from build123d import *

# Parameters (mm, degrees)
F0_W     = 380
F0_H     = 380
F1_DEPTH = 350
F2_W     = 342
F2_H     = 312
F3_DEPTH = 316
F4_W     = 40
F4_H     = 40
F5_DEPTH = 150


with BuildPart() as f1:
    # F0 (on Top) → F1 (new body)
    with BuildSketch(Plane.XY):
        Rectangle(F0_W, F0_H)
    extrude(amount=F1_DEPTH)

    # F2 (on face) → F3 (cut)
    with BuildSketch(Plane.XZ.offset(190)):
        with Locations((0, 175)):
            Rectangle(F2_W, F2_H)
    extrude(amount=-F3_DEPTH, mode=Mode.SUBTRACT)

    # F4 (on face) → F5 (join)
    with BuildSketch(Plane(origin=(0, 0, 0), x_dir=(1, 0, 0), z_dir=(0, 0, -1))):
        with Locations((170, 170)):
            Rectangle(F4_W, F4_H)
        with Locations((-170, -170)):
            Rectangle(F4_W, F4_H)
        with Locations((170, -170)):
            Rectangle(F4_W, F4_H)
        with Locations((-170, 170)):
            Rectangle(F4_W, F4_H)
    extrude(amount=F5_DEPTH)


solid = f1.part
The listing builds one solid part. Answer for the finished solid, in the listing's coordinates (mm). A direction names the side the tool comes from. Give positions to 0.01 mm unless a question says otherwise; leave off trailing zeros. Write each loop counter-clockwise with the first axis right and the second up, starting at its lowest first coordinate (ties: lowest second). Pieces come first, ordered by that corner, then holes. Notation, with made-up numbers: (70, -1) -> (107, -1) arc R11 ccw to (107, 14) -> close; hole circle Ø3 at (41.5, 58.25). An arc over 180 degrees is marked (long way). Use a Markdown table: item, result.
(1) Section C-C, the plane z = 247 is taken. Determine the outline of the cut face in (x, y), then the cut area to 3 significant figures.
Return value:
| item | result |
|---|---|
| outline | (-190, -190) -> (-171, -190) -> (-171, 126) -> (171, 126) -> (171, -190) -> (190, -190) -> (190, 190) -> (-190, 190) -> close |
| area | 36,300 mm2 |
(2) Determine the mould class of faces 6 (the flat face through (-170, -150, -74)), 7 (the flat face through (-170, 150, -74)), 8 (the flat face through (-190, -3, 152)), 9 (the flat face through (-3, 190, 152)) for opening direction Y: released by +Y, released by -Y, zero draft, split by the parting line, or undercut.
Return value:
| item | result |
|---|---|
| face 6 | undercut |
| face 7 | undercut |
| face 8 | zero draft |
| face 9 | released by +Y |
(3) A flat-ended cylindrical pin translates along its axis: P1, Ø6, axis at x = 33.5, y = 118.5, coming from the -Z side. Find the tip coordinate at first contact, or state that the pin passes through.
Return value:
| item | result |
|---|---|
| P1 | z = 0 |
(4) Find the intervals of material crossed by probe 1 along X at (y, z) = (-19, 20); probe 2 along Z at (x, y) = (-3.5, -5.5); probe 3 along Y at (x, z) = (-101.5, 327.5), in increasing order. Write a range as from..to.
Return value:
| item | result |
|---|---|
| probe 1 | -190..-171, 171..190 |
| probe 2 | 0..19, 331..350 |
| probe 3 | 126..190 |
(5) For faces 1 (the flat face through (170, 150, -74)), 2 (the flat face through (150, 170, -74)), 3 (the flat face through (-15, -190, 9)), 4 (the flat face through (-170, 170, -150)), 5 (the flat face through (-171, -34, 173)), determine the directions among +Z, -Z, +X, -X, +Y, -Y from which every point of the face is accessible in a straight line to the end or side of a thin tool.
Return value:
| item | result |
|---|---|
| face 1 | -Z, +X, -X |
| face 2 | -Z, +Y, -Y |
| face 3 | +Z, -Z, +X, -X, -Y |
| face 4 | -Z, +X, -X, +Y, -Y |
| face 5 | -Y |
(6) Section B-B, the plane y = -94 is taken. Determine the outline of the cut face in (x, z), then the cut area to 3 significant figures.
Return value:
| item | result |
|---|---|
| outline | (-190, 0) -> (190, 0) -> (190, 350) -> (-190, 350) -> close; hole (-171, 19) -> (171, 19) -> (171, 331) -> (-171, 331) -> close |
| area | 26,300 mm2 |
(7) Section A-A, the plane z = -106.5 is taken. Determine the outline of the cut face in (x, y), then the cut area to 3 significant figures.
Return value:
| item | result |
|---|---|
| outline | (-190, -190) -> (-150, -190) -> (-150, -150) -> (-190, -150) -> close; (-190, 150) -> (-150, 150) -> (-150, 190) -> (-190, 190) -> close; (150, -190) -> (190, -190) -> (190, -150) -> (150, -150) -> close; (150, 150) -> (190, 150) -> (190, 190) -> (150, 190) -> close |
| area | 6,400 mm2 |
(8) Section D-D, the plane x = -73 is taken. Determine the outline of the cut face in (y, z), then the cut area to 3 significant figures.
Return value:
| item | result |
|---|---|
| outline | (-190, 0) -> (190, 0) -> (190, 350) -> (-190, 350) -> (-190, 331) -> (126, 331) -> (126, 19) -> (-190, 19) -> close |
| area | 34,400 mm2 |
